from build123d import *

# Parameters (mm, degrees)
BOSS_EXTRUDE1_DEPTH  = 6.25
FILLET1_R            = 2
FILLET2_R            = 7
FILLET3_R            = 2
M4_CLEARANCE_HOLE1_D = 4.5


with BuildPart() as part:
    # Sketch1 → Boss-Extrude1 (new body, symmetric)
    with BuildSketch(Plane.XY):
        Polygon((-15.8, 0), (-20.8, 0), (-20.8, 25), (20.8, 25), (20.8, 0), (15.8, 0), (15.8, 20), (-15.8, 20), align=None)
    extrude(amount=BOSS_EXTRUDE1_DEPTH, both=True)

    # Fillet1
    fillet1_edges = [part.edges().sort_by_distance(p)[0] for p in [
        (15.8, 20, 0),
        (-15.8, 20, 0),
    ]]
    fillet(fillet1_edges, radius=FILLET1_R)

    # Fillet2
    fillet2_edges = [part.edges().sort_by_distance(p)[0] for p in [
        (-20.8, 25, 0),
        (20.8, 25, 0),
    ]]
    fillet(fillet2_edges, radius=FILLET2_R)

    # Fillet3
    fillet3_edges = [part.edges().sort_by_distance(p)[0] for p in [
        (18.3, 0, -6.25),
        (18.3, 0, 6.25),
        (-18.3, 0, 6.25),
        (-18.3, 0, -6.25),
    ]]
    fillet(fillet3_edges, radius=FILLET3_R)

    # M4 Clearance Hole1 (through all)
    with Locations(Plane.ZY.offset(20.8)):
        with Locations((0, 7)):
            Hole(M4_CLEARANCE_HOLE1_D / 2)


solid = part.part
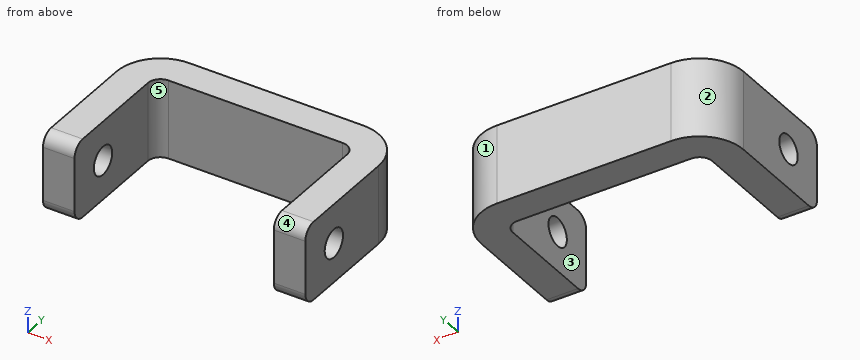
The listing builds one solid part. Answer for the finished solid, in the listing's coordinates (mm). Face numbers are marked on the shaded views. A direction names the side the tool comes from. Give positions to 0.01 mm unless a question says otherwise; leave off trailing zeros. Loops run counter-clockwise (first coordinate to the right, second up) from the corner with the lowest first, then second, coordinate; pieces in that order, holes last.
Item 1: This flat-tipped pin is pushed along its axis until it touches: pin 1 Ø6 at (x, z) = (1.5, -0.5) entering from -Y. Where does it stop, or does it pass through?
Derived:
pin 1: stops at y = 20
Item 2: Determine the mould class of the marked faces 1, 2 and 3 for opening direction X: +X half, -X half, draft (parallel to the pull), parting line (faces both ways), or undercut.
Derived:
face 1: +X half
face 2: -X half
face 3: undercut
Item 3: A cutting plane is placed at C-C (z = 0). Give the vertices of the cut face in (x, y), then the cut area to 3 significant figures.
Derived:
outline: (-20.8, 0) - (-15.8, 0) - (-15.8, 4.75) - (-20.8, 4.75) - close; (-20.8, 9.25) - (-15.8, 9.25) - (-15.8, 18) arc R2 cw to (-13.8, 20) - (13.8, 20) arc R2 cw to (15.8, 18) - (15.8, 9.25) - (20.8, 9.25) - (20.8, 18) arc R7 ccw to (13.8, 25) - (-13.8, 25) arc R7 ccw to (-20.8, 18) - close; (15.8, 0) - (20.8, 0) - (20.8, 4.75) - (15.8, 4.75) - close
area: 344 mm2
Item 4: A cutting plane is placed at B-B (y = 12.5). Give the vertices of the cut face in (x, z).
Derived:
outline: (-20.8, -6.25) - (-15.8, -6.25) - (-15.8, 6.25) - (-20.8, 6.25) - close; (15.8, -6.25) - (20.8, -6.25) - (20.8, 6.25) - (15.8, 6.25) - close
Item 5: A cutting plane is placed at D-D (z = 2.75). Give the vertices of the cut face in (x, y).
Derived:
outline: (-20.8, 0) - (-15.8, 0) - (-15.8, 18) arc R2 cw to (-13.8, 20) - (13.8, 20) arc R2 cw to (15.8, 18) - (15.8, 0) - (20.8, 0) - (20.8, 18) arc R7 ccw to (13.8, 25) - (-13.8, 25) arc R7 ccw to (-20.8, 18) - close
Item 6: A cutting plane is placed at A-A (y = 7). Give the vertices of the cut face in (x, z), then the cut area to 3 significant figures.
Derived:
outline: (-20.8, -6.25) - (-15.8, -6.25) - (-15.8, -2.25) - (-20.8, -2.25) - close; (-20.8, 2.25) - (-15.8, 2.25) - (-15.8, 6.25) - (-20.8, 6.25) - close; (15.8, -6.25) - (20.8, -6.25) - (20.8, -2.25) - (15.8, -2.25) - close; (15.8, 2.25) - (20.8, 2.25) - (20.8, 6.25) - (15.8, 6.25) - close
area: 80.0 mm2
Item 7: Find the intervals of material crossed by line 1 along X through (y, z) = (9.75, -5); line 2 along Y through (x, z) = (1.5, 4.5); line 3 along Y through (x, z) = (-18.75, 0), in increasing order.
Derived:
line 1: x = -20.8 to -15.8, 15.8 to 20.8
line 2: y = 20 to 25
line 3: y = 0 to 4.75, 9.25 to 22.95
Item 8: A tool of negligible diameter and unlimited length cuts with its end or side. For the marked faces 4 and 5, from which of +Z, -Z, +X, -X, +Y, -Y can it reach the whole face along a straight path? Write none if from no direction.
Derived:
face 4: +Z, +X, -X, -Y
face 5: +Z, -Z, -Y
